Design review of the part built by this model. Coordinates are the model's own, in mm. A direction names the side the tool comes from. Coordinates: 2 decimals unless noted, no trailing zeros. Order: outer loops, then holes, each group sorted by start corner. A loop starts at its lowest first (then second) coordinate and runs counter-clockwise, first axis right, second up. Notation, with made-up numbers: M 30.25,73 L 78.25,73 A7 ccw 78.25,77 Z; hole C 62,86.25 d11. An arc over 180 degrees is marked long. Use CSV: the item, a comma, the result in double quotes.
```python
from build123d import *

# Parameters (mm, degrees)
SKETCH1_W                       = 104.5
SKETCH1_H                       = 59.5
BOSS_EXTRUDE1_DEPTH             = 10
BOSS_EXTRUDE2_REACH             = 62.952
BOSS_EXTRUDE2_DIRECTION_2_REACH = 62.952
SKETCH4_W                       = 20
SKETCH4_H                       = 8.5
CUT_EXTRUDE1_DEPTH              = 66.116242213
M4_CLEARANCE_HOLE1_D            = 4.8


with BuildPart() as part:
    # Sketch1 → Boss-Extrude1 (new body)
    with BuildSketch(Plane(origin=(0, 0, 0), x_dir=(1, 0, 0), z_dir=(0, 1, 0))):
        Rectangle(SKETCH1_W, SKETCH1_H)
    extrude(amount=BOSS_EXTRUDE1_DEPTH)

    # Boss-Extrude2: up to this face of the body (flat: up to its plane)
    boss_extrude2_end = Plane(part.part.faces().sort_by_distance((0, 5, 29.75))[0])
    # Sketch3 → Boss-Extrude2 (add, up to the picked face)
    with BuildSketch(Plane.XY, mode=Mode.PRIVATE) as boss_extrude2_sk1:
        with BuildLine():
            Line((52.25, 10), (52.25, 25))
            ThreePointArc((52.25, 25), (42.25, 35), (32.25, 25))
            Line((32.25, 25), (32.25, 10))
            Line((32.25, 10), (52.25, 10))
        make_face()
    boss_extrude2_tool1 = split(extrude(boss_extrude2_sk1.sketch, amount=BOSS_EXTRUDE2_REACH, mode=Mode.PRIVATE), bisect_by=boss_extrude2_end, keep=Keep.BOTH, mode=Mode.PRIVATE)
    add(boss_extrude2_tool1.solids().sort_by(Axis((42.25, 21.535979, 0), (0, 0, 1)))[0])

    # Boss-Extrude2 direction 2: up to this face of the body (flat: up to its plane)
    boss_extrude2_direction_2_end = Plane(part.part.faces().sort_by_distance((0, 5, -29.75))[0])
    # Sketch3 → Boss-Extrude2 direction 2 (add, up to the picked face)
    with BuildSketch(Plane.XY, mode=Mode.PRIVATE) as boss_extrude2_direction_2_sk1:
        with BuildLine():
            Line((52.25, 10), (52.25, 25))
            ThreePointArc((52.25, 25), (42.25, 35), (32.25, 25))
            Line((32.25, 25), (32.25, 10))
            Line((32.25, 10), (52.25, 10))
        make_face()
    boss_extrude2_direction_2_tool1 = split(extrude(boss_extrude2_direction_2_sk1.sketch, amount=-BOSS_EXTRUDE2_DIRECTION_2_REACH, mode=Mode.PRIVATE), bisect_by=boss_extrude2_direction_2_end, keep=Keep.BOTH, mode=Mode.PRIVATE)
    add(boss_extrude2_direction_2_tool1.solids().sort_by(Axis((42.25, 21.535979, 0), (0, 0, -1)))[0])

    # Sketch4 → Cut-Extrude1 (cut, through all)
    with BuildSketch(Plane(origin=(0, 10, 0), x_dir=(1, 0, 0), z_dir=(0, 1, 0))):
        with Locations((42.25, 17)):
            Rectangle(SKETCH4_W, SKETCH4_H)
        with Locations((42.25, 0)):
            Rectangle(SKETCH4_W, SKETCH4_H)
        with Locations((42.25, -17)):
            Rectangle(SKETCH4_W, SKETCH4_H)
    extrude(amount=CUT_EXTRUDE1_DEPTH, mode=Mode.SUBTRACT)

    # M4 Clearance Hole1 (through all)
    with Locations(Plane.XY.offset(29.75)):
        with Locations((42.25, 25)):
            Hole(M4_CLEARANCE_HOLE1_D / 2)


solid = part.part
```
(1) Add section A-A on x = 42.25. Give the number of separate pieces and of enclosed holes in the cut face, and give its area (3 significant figures).
The answers:
separate pieces,"5"
enclosed holes,"0"
area,"1,280 mm2"
(2) Wall thickness on probe 1 along Z at (x, y) = (48.5, 29); probe 2 along Y at (x, z) = (42.25, 26); probe 3 along Y at (x, z) = (3.5, 10): over which ranges is each line inside the solid? List them lowest first.
The answers:
probe 1,"z = -29.75 to -21.25, -12.75 to -4.25, 4.25 to 12.75, 21.25 to 29.75"
probe 2,"y = 0 to 22.6, 27.4 to 35"
probe 3,"y = 0 to 10"
(3) Add section D-D on z = 18. State the section outline as (x, y) points.
The answers:
outline,"M -52.25,0 L 52.25,0 L 52.25,10 L -52.25,10 Z"
(4) Clearance check with flat-ended pins moving along their axes: P1, Ø2.5, axis at y = 17.5, z = 27, coming from the -X side; P2, Ø5, axis at x = 24, z = -23, coming from the -Y side; P3, Ø18, axis at x = -16, z = -7, coming from the +Y side. State where each tip first meets the part, or that it passes through.
The answers:
P1,"stops at x = 32.25"
P2,"stops at y = 0"
P3,"stops at y = 10"
(5) Add section B-B on y = 16.5. State the section outline as (x, z) points.
The answers:
outline,"M 32.25,-29.75 L 52.25,-29.75 L 52.25,-21.25 L 32.25,-21.25 Z; M 32.25,-12.75 L 52.25,-12.75 L 52.25,-4.25 L 32.25,-4.25 Z; M 32.25,4.25 L 52.25,4.25 L 52.25,12.75 L 32.25,12.75 Z; M 32.25,21.25 L 52.25,21.25 L 52.25,29.75 L 32.25,29.75 Z"
(6) Add section C-C on x = -42. State the section outline as (y, z) points.
The answers:
outline,"M 0,-29.75 L 10,-29.75 L 10,29.75 L 0,29.75 Z"
(7) The part is to be moulded in two halves that separate along Y. For faces 1 (the face through (42.77, 22.657, 8.441)), 2 (the face through (32.25, 18, 26)), 3 (the face through (42.47, 34.998, -25.44)), say which applies: pulls with the +Y half, pulls with the -Y half, needs draft (parallel to the pull), parting line crosses it, or undercut.
The answers:
face 1,"undercut"
face 2,"needs draft"
face 3,"pulls with the +Y half"
(8) For faces 4 (the face through (-1, 10, 0)), 5 (the face through (32.25, 18, -25)), 6 (the face through (42, 22, 4.25)), list the 3-axis set-ups (+Z, -Z, +X, -X, +Y, -Y) from which the entire face can be reached by the end or side of a thin tool; tool diameter is ignored.
The answers:
face 4,"-X, +Y"
face 5,"+Z, -Z, -X, +Y"
face 6,"+X, -X, +Y"
